```python
from build123d import *

# Parameters (mm, degrees)
SKETCH1_W           = 21
SKETCH1_H           = 15.4
BOSS_EXTRUDE1_DEPTH = 15.1
SKETCH3_W           = 21
SKETCH3_H           = 15.1
SKETCH3_W_2         = 18.7
SKETCH3_H_2         = 13
CUT_EXTRUDE1_DEPTH  = 13.4
SKETCH4_W           = 18
SKETCH4_H           = 10
BOSS_EXTRUDE2_DEPTH = 3
CUT_EXTRUDE2_DEPTH  = 13.55


with BuildPart() as part:
    # Sketch1 → Boss-Extrude1 (new body)
    with BuildSketch(Plane.XY):
        with Locations((10.5, -7.7)):
            Rectangle(SKETCH1_W, SKETCH1_H)
    extrude(amount=BOSS_EXTRUDE1_DEPTH)

    # Sketch3 → Cut-Extrude1 (cut)
    with BuildSketch(Plane(origin=(0, 0, 0), x_dir=(1, 0, 0), z_dir=(0, 1, 0))):
        with Locations((10.5, -7.55)):
            Rectangle(SKETCH3_W, SKETCH3_H)
        with Locations((10.5, -7.55)):
            Rectangle(SKETCH3_W_2, SKETCH3_H_2, mode=Mode.SUBTRACT)
    extrude(amount=-CUT_EXTRUDE1_DEPTH, mode=Mode.SUBTRACT)

    # Sketch4 → Boss-Extrude2 (add)
    with BuildSketch(Plane.XZ.offset(15.4)):
        with Locations((10.5, 7.55)):
            Rectangle(SKETCH4_W, SKETCH4_H)
    extrude(amount=BOSS_EXTRUDE2_DEPTH)

    # Sketch5 → Cut-Extrude2 (cut, through all)
    with BuildSketch(Plane(origin=(0, 0, 2.55), x_dir=(-1, 0, 0), z_dir=(0, 0, -1))):
        with BuildLine():
            Line((-4.318187888, -15.4), (-5.64025516, -18.208957591))
            ThreePointArc((-5.64025516, -18.208957591), (-5.758218198, -18.313607167), (-5.91534374, -18.300251418))
            add(Edge.make_bspline(
                [(-5.91534374, -18.300251418), (-9.414175538, -16.433895122), (-13.180982291, -15.465516785), (-17.200671876, -15.4)],
                knots=[0.017358171, 0.017358171, 0.017358171, 0.017358171, 1, 1, 1, 1], degree=3))
            Line((-17.200671876, -15.4), (-19.5, -15.4))
            Line((-19.5, -15.4), (-20.228637612, -15.606353341))
            Line((-20.228637612, -15.606353341), (-20.675659597, -18.662431802))
            Line((-20.675659597, -18.662431802), (-18.82613024, -20.157147076))
            Line((-18.82613024, -20.157147076), (-11.911793742, -20.360373848))
            Line((-11.911793742, -20.360373848), (-0.335637878, -21.060292332))
            Line((-0.335637878, -21.060292332), (-0.808442559, -15.4))
            Line((-0.808442559, -15.4), (-4.318187888, -15.4))
        make_face()
    extrude(amount=-CUT_EXTRUDE2_DEPTH, mode=Mode.SUBTRACT)


solid = part.part
```
The model under review builds one solid part; all positions refer to its coordinate system, in mm. A direction names the side the tool comes from. Coordinates: 2 decimals unless noted, no trailing zeros. Write each loop counter-clockwise with the first axis right and the second up, starting at its lowest first coordinate (ties: lowest second). Pieces come first, ordered by that corner, then holes. Notation, with made-up numbers: (37, 46) - (69, 46) arc R15 ccw to (69, 53) - close; hole circle Ø4 at (-12, -21.75). An arc over 180 degrees is marked (long way). Write item = value, one per line.
(1) Consider section A-A, the plane z = 13.25. Give the boundary of the cut face in (x, y), then the cut area to 3 significant figures.
Result sheet:
outline = (0, -15.4) - (21, -15.4) - (21, -13.4) - (19.85, -13.4) - (19.85, 0) - (1.15, 0) - (1.15, -13.4) - (0, -13.4) - close
area = 293 mm^2
(2) Machinability: for faces 1 (the face through (8, -16, 12.55)), 2 (the face through (10, -7, 14.05)), 3 (the face through (19.85, -7, 8)), 4 (the face through (8, -16, 2.55)), which of the approach directions +Z, -Z, +X, -X, +Y, -Y give a long, thin tool a straight path to every point of the face, cutting with its end or side? Answer none if there is none.
Result sheet:
face_1 = +Z, +X, -X, -Y
face_2 = +Z, +X, -X, +Y
face_3 = +Z, -Z, +X, +Y
face_4 = -Z, +X, -X, -Y
(3) Consider section C-C, the plane y = -12.75. Give the boundary of the cut face in (x, z).
Result sheet:
outline = (1.15, 1.05) - (19.85, 1.05) - (19.85, 14.05) - (1.15, 14.05) - close
(4) For P1, Ø8, axis at y = -2, z = 5.5, coming from the -X side; P2, Ø8, axis at y = -2.5, z = 9.5, coming from the +X side; P3, Ø4, axis at x = 7.5, z = 10, coming from the +Y side; P4, Ø0.9, axis at x = 11, y = -16.5, coming from the -Z side, all flat-tipped, find the tip position at first contact; note any pin that passes through.
Result sheet:
P1 = 1.15
P2 = 19.85
P3 = 0
P4 = 2.55
(5) Consider section B-B, the plane x = 3.25. Give the boundary of the cut face in (y, z), then the cut area to 3 significant figures.
Result sheet:
outline = (-15.4, 0) - (-13.4, 0) - (-13.4, 1.05) - (0, 1.05) - (0, 14.05) - (-13.4, 14.05) - (-13.4, 15.1) - (-15.4, 15.1) - close
area = 204 mm^2
(6) For line 1 (X direction, y = -10, z = 9.5); line 2 (Z direction, x = 17.5, y = -9.25); line 3 (Y direction, x = 17.25, z = 14.75), list the stretches that pass through material, from the lowest coordinate up. Write a range as [from, to].
Result sheet:
line_1 = [1.15, 19.85]
line_2 = [1.05, 14.05]
line_3 = [-15.4, -13.4]
